```python
from build123d import *

# Parameters (mm, degrees)
SKETCH1_W              = 54
SKETCH1_H              = 300
BOSS_EXTRUDE1_DEPTH    = 6.35
FILLET1_R              = 5
SKETCH3_R              = 5
CUT_EXTRUDE1_DEPTH     = 7.35
F_6_CLEARANCE_HOLE1_D  = 3.6576
SKETCH6_W              = 33.65
SKETCH6_H              = 6.35
CUT_EXTRUDE2_DEPTH     = 7.35
F_10_CLEARANCE_HOLE2_D = 4.9784


with BuildPart() as part:
    # Sketch1 → Boss-Extrude1 (new body)
    with BuildSketch(Plane.XY):
        Rectangle(SKETCH1_W, SKETCH1_H)
    extrude(amount=BOSS_EXTRUDE1_DEPTH)

    # Fillet1
    fillet1_edges = [part.edges().sort_by_distance(p)[0] for p in [
        (-27, -150, 3.175),
        (-27, 150, 3.175),
        (27, 150, 3.175),
        (27, -150, 3.175),
    ]]
    fillet(fillet1_edges, radius=FILLET1_R)

    # Sketch3 → Cut-Extrude1 (cut, through all)
    with BuildSketch(Plane.XY.offset(6.35)):
        with Locations((0, 82.5)):
            Circle(SKETCH3_R)
    extrude(amount=-CUT_EXTRUDE1_DEPTH, mode=Mode.SUBTRACT)

    # #6 Clearance Hole1 (through all)
    with Locations(Plane.XY.offset(6.35)):
        with Locations((-22, 104.5), (-22, 60.5), (22, 60.5), (22, 104.5), (-1.944797213, 123.085202787), (-1.944797213, 136.914797213), (11.884797213, 136.914797213), (11.884797213, 123.085202787), (-1.944797213, 41.914797213), (11.884797213, 41.914797213), (11.884797213, 28.085202787), (-1.944797213, 28.085202787)):
            Hole(F_6_CLEARANCE_HOLE1_D / 2)

    # Sketch6 → Cut-Extrude2 (cut, through all)
    with BuildSketch(Plane.XY.offset(6.35)):
        with Locations((0, -140.475)):
            Rectangle(SKETCH6_W, SKETCH6_H)
    extrude(amount=-CUT_EXTRUDE2_DEPTH, mode=Mode.SUBTRACT)

    # #10 Clearance Hole2 (through all)
    with Locations(Plane.XY.offset(6.35)):
        with Locations((0, 64.25), (0, 100.75)):
            Hole(F_10_CLEARANCE_HOLE2_D / 2)


solid = part.part
```
The listing builds one solid part. Answer for the finished solid, in the listing's coordinates (mm). A direction names the side the tool comes from. Give positions to 0.01 mm unless a question says otherwise; leave off trailing zeros. Loops run counter-clockwise (first coordinate to the right, second up) from the corner with the lowest first, then second, coordinate; pieces in that order, holes last. Notation, with made-up numbers: (39, 69) - (96, 69) arc R10 ccw to (96, 88) - close; hole circle Ø2 at (-4.5, 13.5). An arc over 180 degrees is marked (long way). Return JSON: item names as keys, results as strings. Group by question number.
1. Given pin 1 Ø3 at (x, y) = (11.88, 123.09) entering from -Z; pin 2 Ø6 at (x, y) = (-1.94, 28.09) entering from +Z, each flat-ended and moving along its own axis, determine where each tip first touches the part or whether it passes through.
2. Find section B-B (z = 2). State how many separate pieces and enclosed holes the cut face has, then the cut area to 3 significant figures.
3. Determine the mould class of faces 1 (the cylindrical face through (0.32, 103.22, 3.13)), 2 (the flat face through (27, -2, 3)), 3 (the flat face through (-27, -2, 3)) for opening direction X: pulls with the +X half, pulls with the -X half, needs draft (parallel to the pull), parting line crosses it, or undercut.
4. Which of the six approach directions +Z, -Z, +X, -X, +Y, -Y give full straight-line access (tool end or side, diameter ignored) to faces 4 (the flat face through (0, -143.65, 3)), 5 (the cylindrical face through (-26, 148, 3))?
5. Straight lines are drawn through the part: line 1 (Y direction, x = 11.5, z = 1.75); line 2 (X direction, y = 104.5, z = 1.5); line 3 (Y direction, x = 0, z = 4). For each, find the intervals that lie inside material, in ascending order. Write a range as [from, to].
6. Find section A-A (y = 82.5). Write down the section's boundary in (x, z), then the cut area to 3 significant figures.
Verdict:
{
 "1": {"pin 1": "passes through", "pin 2": "stops at z = 6.35"},
 "2": {"separate pieces": "1", "enclosed holes": "16", "area": "15,700 mm^2"},
 "3": {"face 1": "undercut", "face 2": "pulls with the +X half", "face 3": "pulls with the -X half"},
 "4": {"face 4": "+Z, -Z", "face 5": "+Z, -Z, -X, +Y"},
 "5": {"line 1": "y = [-150, -143.65], [-137.3, 26.3], [29.87, 40.13], [43.7, 121.3], [124.87, 135.13], [138.7, 150]", "line 2": "x = [-27, -23.83], [-20.17, 20.17], [23.83, 27]", "line 3": "y = [-150, -143.65], [-137.3, 61.76], [66.74, 77.5], [87.5, 98.26], [103.24, 150]"},
 "6": {"outline": "(-27, 0) - (-5, 0) - (-5, 6.35) - (-27, 6.35) - close; (5, 0) - (27, 0) - (27, 6.35) - (5, 6.35) - close", "area": "279 mm^2"}
}
